Source: CAD feature listing. Evaluate the final solid. Frame: model axes, mm. Face numbers are marked on the shaded views. Round coordinates to 2 decimals unless told otherwise and drop trailing zeros. Loops run counter-clockwise (first coordinate to the right, second up) from the corner with the lowest first, then second, coordinate; pieces in that order, holes last.
Item 1: First-contact query: P1, Ø2.5, axis at x = -38, z = 8.5, coming from the -Y side; P2, Ø2, axis at x = -23.53, y = 31.25, coming from the -Z side; P3, Ø4, axis at x = -45, z = 11.5, coming from the -Y side; P4, Ø5, axis at y = -17.5, z = 12, coming from the -X side. Flat tips, straight axial feed; report the tip coordinate or a pass-through.
Item 2: Ray query, L1, parallel to Y at x = -40, z = 8; L2, parallel to Z at x = -36, y = 9; L3, parallel to Y at x = -31, z = 9.25. Return the intervals inside material, ascending.
Item 3: Section query A-A on y = 6.98. Return loops of the section in (x, z), then the cut area to 3 significant figures.
Item 4: Section query D-D on x = -45. Return loops of the section in (y, z).
Item 5: Pull-direction query (Y, two-part tool) for the marked faces 1 and 2; classes: released by +Y, released by -Y, zero draft, split by the parting line, or undercut.
Item 6: Section query B-B on z = 13. Return loops of the section in (x, y).
Item 7: Section query C-C on x = -24. Return loops of the section in (y, z).
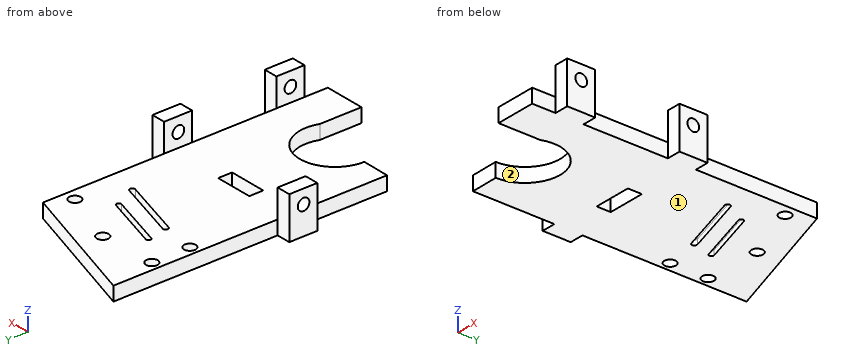
```python
from build123d import *

# Parameters (mm, degrees)
SKETCH1_W            = 29.13
SKETCH1_H            = 2
BOSS_EXTRUDE1_DEPTH  = 45.22
SKETCH15_W           = 3.835
SKETCH15_H           = 2
BOSS_EXTRUDE7_DEPTH  = 25.02
SKETCH19_W           = 2
SKETCH19_H           = 6
BOSS_EXTRUDE9_DEPTH  = 3
SKETCH20_W           = 3
SKETCH20_H           = 6
BOSS_EXTRUDE10_DEPTH = 6
CUT_EXTRUDE10_DEPTH  = 4
SKETCH27_R           = 1.25
CUT_EXTRUDE13_DEPTH  = 5
CUT_EXTRUDE16_DEPTH  = 4.86
CUT_EXTRUDE20_DEPTH  = 5
SKETCH28_R           = 1.25
CUT_EXTRUDE23_DEPTH  = 5
SKETCH32_R           = 1.25
CUT_EXTRUDE25_DEPTH  = 5
SKETCH38_W           = 2
SKETCH38_H           = 6
BOSS_EXTRUDE11_DEPTH = 3
SKETCH39_W           = 3
SKETCH39_H           = 6
BOSS_EXTRUDE12_DEPTH = 6
SKETCH40_R           = 1.250000005
CUT_EXTRUDE26_DEPTH  = 6
SKETCH51_W           = 2
SKETCH51_H           = 6
BOSS_EXTRUDE15_DEPTH = 3
SKETCH52_W           = 3
SKETCH52_H           = 6
BOSS_EXTRUDE16_DEPTH = 6
SKETCH53_R           = 1.249999995
CUT_EXTRUDE28_DEPTH  = 6
SKETCH54_R           = 1.25
CUT_EXTRUDE29_DEPTH  = 3
CUT_EXTRUDE30_DEPTH  = 10
BOSS_EXTRUDE17_DEPTH = 3
SKETCH57_R           = 1.25
BOSS_EXTRUDE18_DEPTH = 1
SKETCH58_W           = 8
SKETCH58_H           = 3
CUT_EXTRUDE31_DEPTH  = 10


with BuildPart() as part:
    # Sketch1 → Boss-Extrude1 (new body)
    with BuildSketch(Plane(origin=(0, 0, 0), x_dir=(1, 0, 0), z_dir=(0, 1, 0))):
        with Locations((-35.580481579, -22.688974349)):
            Rectangle(SKETCH1_W, SKETCH1_H)
    extrude(amount=BOSS_EXTRUDE1_DEPTH)

    # Sketch15 → Boss-Extrude7 (add)
    with BuildSketch(Plane.XZ):
        with Locations((-22.932981579, 22.688974349)):
            Rectangle(SKETCH15_W, SKETCH15_H)
    extrude(amount=BOSS_EXTRUDE7_DEPTH)

    # Sketch19 → Boss-Extrude9 (add)
    with BuildSketch(Plane(origin=(-21.015481579, 0, 0), x_dir=(0, 0, -1), z_dir=(1, 0, 0))):
        with Locations((-22.688974349, -17.02)):
            Rectangle(SKETCH19_W, SKETCH19_H)
    extrude(amount=BOSS_EXTRUDE9_DEPTH)

    # Sketch20 → Boss-Extrude10 (add)
    with BuildSketch(Plane(origin=(0, 0, 21.688974349), x_dir=(-1, 0, 0), z_dir=(0, 0, -1))):
        with Locations((19.515481579, -17.02)):
            Rectangle(SKETCH20_W, SKETCH20_H)
    extrude(amount=BOSS_EXTRUDE10_DEPTH)

    # Sketch24 → Cut-Extrude10 (cut)
    with BuildSketch(Plane.XY.offset(23.688974349)):
        Polygon((-21.015481579, 45.22), (-21.015481579, 37.57), (-50.145481579, 45.22), align=None)
    extrude(amount=-CUT_EXTRUDE10_DEPTH, mode=Mode.SUBTRACT)

    # Sketch27 → Cut-Extrude13 (cut)
    with BuildSketch(Plane.XY.offset(23.688974349)):
        with Locations((-48.155481573, 35.325814089)):
            Circle(SKETCH27_R)
        with Locations((-48.155481573, 27.181192799)):
            Circle(SKETCH27_R)
    extrude(amount=-CUT_EXTRUDE13_DEPTH, mode=Mode.SUBTRACT)

    # Sketch35 → Cut-Extrude16 (cut)
    with BuildSketch(Plane.XY.offset(23.688974349)):
        Polygon((-21.015481579, 35.99), (-21.015481579, 37.57), (-50.145481579, 45.22), align=None)
    extrude(amount=-CUT_EXTRUDE16_DEPTH, mode=Mode.SUBTRACT)


with BuildPart() as body_2:
    # Mirror1: mirrored copy
    add(part.part.mirror(Plane(origin=(0, 0, 15.688974349), x_dir=(1, 0, 0), z_dir=(0, 0, -1))))

    # Sketch37 → Cut-Extrude20 (cut)
    with BuildSketch(Plane(origin=(0, 0, 7.688974349), x_dir=(-1, 0, 0), z_dir=(0, 0, -1))):
        with BuildLine():
            Line((29.422391304, 27.369440111), (41.452993211, 31.026802565))
            ThreePointArc((41.452993211, 31.026802565), (42.065476612, 30.699897808), (41.738571855, 30.087414406))
            Line((41.738571855, 30.087414406), (29.707969948, 26.430051952))
            ThreePointArc((29.707969948, 26.430051952), (29.095486546, 26.75695671), (29.422391304, 27.369440111))
        make_face()
        with BuildLine():
            Line((26.963881394, 22.478846245), (40.405895564, 26.565285004))
            ThreePointArc((40.405895564, 26.565285004), (41.083801623, 26.203461785), (40.721978404, 25.525555725))
            Line((40.721978404, 25.525555725), (27.279964235, 21.439116966))
            ThreePointArc((27.279964235, 21.439116966), (26.602058175, 21.800940185), (26.963881394, 22.478846245))
        make_face()
    extrude(amount=-CUT_EXTRUDE20_DEPTH, mode=Mode.SUBTRACT)


with BuildPart() as body_2_2:
    # Mirror2: mirrored copy
    add(body_2.part.mirror(Plane.XY.offset(15.688974349)))

    # Sketch28 → Cut-Extrude23 (cut)
    with BuildSketch(Plane.XY.offset(23.688974349)):
        with Locations((-23.525481526, 31.253503444)):
            Circle(SKETCH28_R)
    extrude(amount=-CUT_EXTRUDE23_DEPTH, mode=Mode.SUBTRACT)

    # Sketch32 → Cut-Extrude25 (cut)
    with BuildSketch(Plane.XY.offset(23.688974349)):
        with Locations((-36.114456484, 35.789812978)):
            Circle(SKETCH32_R)
    extrude(amount=-CUT_EXTRUDE25_DEPTH, mode=Mode.SUBTRACT)

    # Sketch38 → Boss-Extrude11 (add)
    with BuildSketch(Plane.ZY.offset(50.145481579)):
        with Locations((22.688974349, 7.042669101)):
            Rectangle(SKETCH38_W, SKETCH38_H)
    extrude(amount=BOSS_EXTRUDE11_DEPTH)

    # Sketch39 → Boss-Extrude12 (add)
    with BuildSketch(Plane(origin=(0, 0, 21.688974349), x_dir=(-1, 0, 0), z_dir=(0, 0, -1))):
        with Locations((51.645481579, 7.042669101)):
            Rectangle(SKETCH39_W, SKETCH39_H)
    extrude(amount=BOSS_EXTRUDE12_DEPTH)

    # Sketch40 → Cut-Extrude26 (cut)
    with BuildSketch(Plane.ZY.offset(53.145481579)):
        with Locations((18.688974344, 6.98)):
            Circle(SKETCH40_R)
    extrude(amount=-CUT_EXTRUDE26_DEPTH, mode=Mode.SUBTRACT)

    # Sketch51 → Boss-Extrude15 (add)
    with BuildSketch(Plane(origin=(-21.015481579, 0, 0), x_dir=(0, 0, -1), z_dir=(1, 0, 0))):
        with Locations((-22.688974349, 7.042669101)):
            Rectangle(SKETCH51_W, SKETCH51_H)
    extrude(amount=BOSS_EXTRUDE15_DEPTH)

    # Sketch52 → Boss-Extrude16 (add)
    with BuildSketch(Plane(origin=(0, 0, 21.688974349), x_dir=(-1, 0, 0), z_dir=(0, 0, -1))):
        with Locations((19.515481579, 7.042669101)):
            Rectangle(SKETCH52_W, SKETCH52_H)
    extrude(amount=BOSS_EXTRUDE16_DEPTH)

    # Sketch53 → Cut-Extrude28 (cut)
    with BuildSketch(Plane(origin=(-18.015481579, 0, 0), x_dir=(0, 0, -1), z_dir=(1, 0, 0))):
        with Locations(Location((-18.688974344, 6.98, 0), (0, 0, 180))):
            Circle(SKETCH53_R)
    extrude(amount=-CUT_EXTRUDE28_DEPTH, mode=Mode.SUBTRACT)


with BuildPart() as body_2_3:
    # Mirror4: mirrored copy
    add(body_2_2.part.mirror(Plane(origin=(0, 0, 15.688974349), x_dir=(1, 0, 0), z_dir=(0, 0, -1))))

    # Sketch54 → Cut-Extrude29 (cut)
    with BuildSketch(Plane(origin=(-18.015481579, 0, 0), x_dir=(0, 0, -1), z_dir=(1, 0, 0))):
        with Locations((-12.688974354, -17.012020694)):
            Circle(SKETCH54_R)
    extrude(amount=-CUT_EXTRUDE29_DEPTH, mode=Mode.SUBTRACT)

    # Sketch55 → Cut-Extrude30 (cut)
    with BuildSketch(Plane(origin=(0, 0, 7.688974349), x_dir=(-1, 0, 0), z_dir=(0, 0, -1))):
        Polygon((24.850481579, 0), (21.015481579, -25.02), (24.850481579, -25.02), align=None)
    extrude(amount=-CUT_EXTRUDE30_DEPTH, mode=Mode.SUBTRACT)

    # Sketch56 → Boss-Extrude17 (add)
    with BuildSketch(Plane.XY.offset(9.688974349)):
        with BuildLine():
            Line((-21.015481579, -25.02), (-24.850481579, 0))
            Line((-24.850481579, 0), (-50.145481579, 0))
            Line((-50.145481579, 0), (-50.145481579, -13.39301212))
            Line((-50.145481579, -13.39301212), (-44.248800379, -13.458826151))
            ThreePointArc((-44.248800379, -13.458826151), (-35.383312942, -6.047023199), (-29.659784654, -16.085594533))
            Line((-29.659784654, -16.085594533), (-29.659784654, -25.02))
            Line((-29.659784654, -25.02), (-21.015481579, -25.02))
        make_face()
    extrude(amount=-BOSS_EXTRUDE17_DEPTH)

    # Sketch57 → Boss-Extrude18 (add)
    with BuildSketch(Plane(origin=(0, 0, 7.688974349), x_dir=(-1, 0, 0), z_dir=(0, 0, -1))):
        Polygon((21.015481579, -25.02), (21.015481579, -20.02), (18.015481579, -20.02), (18.015481579, -14.02), (21.015481579, -14.02), (21.015481579, 4.042669101), (18.015481579, 4.042669101), (18.015481579, 10.042669101), (21.015481579, 10.042669101), (21.015481579, 35.99), (50.145481579, 45.22), (50.145481579, 10.042669101), (53.145481579, 10.042669101), (53.145481579, 4.042669101), (50.145481579, 4.042669101), (50.145481579, 0), (24.850481579, 0), align=None)
        with Locations(Location((23.525481526, 31.253503444, 0), (0, 0, 180))):
            Circle(SKETCH57_R, mode=Mode.SUBTRACT)
        with Locations(Location((36.114456484, 35.789812978, 0), (0, 0, 180))):
            Circle(SKETCH57_R, mode=Mode.SUBTRACT)
        with Locations(Location((48.155481573, 35.325814089, 0), (0, 0, 180))):
            Circle(SKETCH57_R, mode=Mode.SUBTRACT)
        with Locations(Location((48.155481573, 27.181192799, 0), (0, 0, 180))):
            Circle(SKETCH57_R, mode=Mode.SUBTRACT)
        with BuildLine():
            Line((29.422855642, 27.367912705), (41.45345755, 31.025275159))
            ThreePointArc((41.45345755, 31.025275159), (42.063949206, 30.699433469), (41.738107516, 30.088941812))
            Line((41.738107516, 30.088941812), (29.707505609, 26.431579358))
            ThreePointArc((29.707505609, 26.431579358), (29.097013952, 26.757421048), (29.422855642, 27.367912705))
        make_face(mode=Mode.SUBTRACT)
        with BuildLine():
            Line((26.964038287, 22.478330158), (40.406052456, 26.564768917))
            ThreePointArc((40.406052456, 26.564768917), (41.083285536, 26.203304892), (40.721821511, 25.526071812))
            Line((40.721821511, 25.526071812), (27.279807342, 21.439633053))
            ThreePointArc((27.279807342, 21.439633053), (26.602574262, 21.801097078), (26.964038287, 22.478330158))
        make_face(mode=Mode.SUBTRACT)
    extrude(amount=BOSS_EXTRUDE18_DEPTH)

    # Sketch58 → Cut-Extrude31 (cut)
    with BuildSketch(Plane(origin=(0, 0, 6.688974349), x_dir=(-1, 0, 0), z_dir=(0, 0, -1))):
        with Locations((37.080481579, 7.042669101)):
            Rectangle(SKETCH58_W, SKETCH58_H)
    extrude(amount=-CUT_EXTRUDE31_DEPTH, mode=Mode.SUBTRACT)


solid = body_2_3.part
```
Data:
1. P1: stops at y = -6.37
1. P2: passes through
1. P3: stops at y = -13.46
1. P4: stops at x = -29.66
2. L1: y = -6.68 to 5.54, 8.54 to 25.31, 26.44 to 29.56, 30.59 to 42.01
2. L2: z = 6.69 to 9.69
2. L3: y = -8.56 to 22.57, 23.71 to 26.82, 27.85 to 39.15
3. outline: (-53.15, 6.69) - (-41.08, 6.69) - (-41.08, 9.69) - (-50.15, 9.69) - (-50.15, 11.44) - (-53.15, 11.44) - close; (-53.15, 13.94) - (-50.15, 13.94) - (-50.15, 15.69) - (-53.15, 15.69) - close; (-33.08, 6.69) - (-18.02, 6.69) - (-18.02, 11.44) - (-21.02, 11.44) - (-21.02, 9.69) - (-33.08, 9.69) - close; (-21.02, 13.94) - (-18.02, 13.94) - (-18.02, 15.69) - (-21.02, 15.69) - close
3. area: 102 mm2
4. outline: (-13.45, 6.69) - (43.59, 6.69) - (43.59, 9.69) - (-13.45, 9.69) - close
5. face 1: zero draft
5. face 2: undercut
6. outline: (-53.15, 4.04) - (-50.15, 4.04) - (-50.15, 5.77) - (-53.15, 5.77) - close; (-53.15, 8.19) - (-50.15, 8.19) - (-50.15, 10.04) - (-53.15, 10.04) - close; (-21.02, -20.02) - (-18.02, -20.02) - (-18.02, -18.22) - (-21.02, -18.22) - close; (-21.02, -15.8) - (-18.02, -15.8) - (-18.02, -14.02) - (-21.02, -14.02) - close; (-21.02, 4.04) - (-18.02, 4.04) - (-18.02, 5.77) - (-21.02, 5.77) - close; (-21.02, 8.19) - (-18.02, 8.19) - (-18.02, 10.04) - (-21.02, 10.04) - close
7. outline: (-25.02, 6.69) - (30.1, 6.69) - (30.1, 9.69) - (-25.02, 9.69) - close; (32.41, 6.69) - (36.94, 6.69) - (36.94, 9.69) - (32.41, 9.69) - close
